Source: CAD feature listing. Evaluate the final solid. Frame: model axes, mm. A direction names the side the tool comes from. Give positions to 0.01 mm unless a question says otherwise; leave off trailing zeros. Loops run counter-clockwise (first coordinate to the right, second up) from the corner with the lowest first, then second, coordinate; pieces in that order, holes last. Notation, with made-up numbers: M 22.5,3.25 L 60.5,3.25 A25 ccw 60.5,17.25 Z; hole C 21.5,88.5 d8. An arc over 180 degrees is marked long. Answer in a Markdown table with one row per item.
```python
from build123d import *

# Parameters (mm, degrees)
SKETCH1_W           = 44.1
SKETCH1_H           = 8
BOSS_EXTRUDE1_DEPTH = 2
SKETCH2_W           = 12
SKETCH2_H           = 2
BOSS_EXTRUDE2_DEPTH = 3
CUT_EXTRUDE1_DEPTH  = 46.097782651
SKETCH4_W           = 32.1
SKETCH4_H           = 2
BOSS_EXTRUDE3_DEPTH = 1
SKETCH7_R           = 2.794
CUT_EXTRUDE3_DEPTH  = 45.382541613
SKETCH8_R           = 1.5875
CUT_EXTRUDE4_DEPTH  = 45.382541613
BOSS_EXTRUDE4_DEPTH = 3


with BuildPart() as part:
    # Sketch1 → Boss-Extrude1 (new body)
    with BuildSketch(Plane(origin=(0, 0, 0), x_dir=(1, 0, 0), z_dir=(0, 1, 0))):
        with Locations((22.05, 0)):
            Rectangle(SKETCH1_W, SKETCH1_H)
    boss_extrude1 = extrude(amount=BOSS_EXTRUDE1_DEPTH)

    # Sketch2 → Boss-Extrude2 (add)
    with BuildSketch(Plane(origin=(0, 2, 0), x_dir=(1, 0, 0), z_dir=(0, 1, 0))):
        with Locations((38.1, 3)):
            Rectangle(SKETCH2_W, SKETCH2_H)
        with Locations((38.1, -3)):
            Rectangle(SKETCH2_W, SKETCH2_H)
    boss_extrude2 = extrude(amount=BOSS_EXTRUDE2_DEPTH)

    # Sketch3 → Cut-Extrude1 (cut, through all)
    with BuildSketch(Plane.XY.offset(4)):
        with BuildLine():
            Line((36.6, 3.5), (36.6, 5))
            Line((36.6, 5), (39.6, 5))
            Line((39.6, 5), (39.6, 3.5))
            ThreePointArc((39.6, 3.5), (38.1, 2), (36.6, 3.5))
        make_face()
    cut_extrude1 = extrude(amount=-CUT_EXTRUDE1_DEPTH, mode=Mode.SUBTRACT)

    # Sketch4 → Boss-Extrude3 (add)
    with BuildSketch(Plane(origin=(0, 2, 0), x_dir=(1, 0, 0), z_dir=(0, 1, 0))):
        with Locations((16.05, -3)):
            Rectangle(SKETCH4_W, SKETCH4_H)
        with Locations((16.05, 3)):
            Rectangle(SKETCH4_W, SKETCH4_H)
    boss_extrude3 = extrude(amount=BOSS_EXTRUDE3_DEPTH)

    # Mirror1: Boss-Extrude1, Boss-Extrude2, Cut-Extrude1, Boss-Extrude3 across plane
    add(boss_extrude1.mirror(Plane(origin=(0, 0, 0), x_dir=(0, 0, 1), z_dir=(1, 0, 0))))
    add(boss_extrude2.mirror(Plane(origin=(0, 0, 0), x_dir=(0, 0, 1), z_dir=(1, 0, 0))))
    add(cut_extrude1.mirror(Plane(origin=(0, 0, 0), x_dir=(0, 0, 1), z_dir=(1, 0, 0))), mode=Mode.SUBTRACT)
    add(boss_extrude3.mirror(Plane(origin=(0, 0, 0), x_dir=(0, 0, 1), z_dir=(1, 0, 0))))

    # Sketch7 → Cut-Extrude3 (cut, through all)
    with BuildSketch(Plane(origin=(0, 2, 0), x_dir=(1, 0, 0), z_dir=(0, 1, 0))):
        Circle(SKETCH7_R)
    extrude(amount=CUT_EXTRUDE3_DEPTH, mode=Mode.SUBTRACT)

    # Sketch8 → Cut-Extrude4 (cut, through all)
    with BuildSketch(Plane(origin=(0, 2, 0), x_dir=(1, 0, 0), z_dir=(0, 1, 0))):
        with Locations(Location((0, 0, 0), (0, 0, 270))):
            Circle(SKETCH8_R)
    extrude(amount=-CUT_EXTRUDE4_DEPTH, mode=Mode.SUBTRACT)

    # Sketch9 → Boss-Extrude4 (add)
    with BuildSketch(Plane(origin=(0, 3, 0), x_dir=(1, 0, 0), z_dir=(0, 1, 0))):
        with BuildLine():
            Line((-2.642429942, -4), (2.642429942, -4))
            ThreePointArc((2.642429942, -4), (0, -4.794), (-2.642429942, -4))
        make_face()
        with BuildLine():
            Line((2.642429942, 4), (-2.642429942, 4))
            ThreePointArc((-2.642429942, 4), (0, 4.794), (2.642429942, 4))
        make_face()
    extrude(amount=-BOSS_EXTRUDE4_DEPTH)


solid = part.part
```
1) Section C-C, the plane x = 17. Return loops of the section in (y, z).
Reply:
| item | result |
|---|---|
| outline | M 0,-4 L 3,-4 L 3,-2 L 2,-2 L 2,2 L 3,2 L 3,4 L 0,4 Z |
2) Section A-A, the plane x = 0. Return loops of the section in (y, z), then the cut area to 3 significant figures.
Reply:
| item | result |
|---|---|
| outline | M 0,-4.79 L 3,-4.79 L 3,-2.79 L 2,-2.79 L 2,-1.59 L 0,-1.59 Z; M 0,1.59 L 2,1.59 L 2,2.79 L 3,2.79 L 3,4.79 L 0,4.79 Z |
| area | 16.8 mm² |
3) Section B-B, the plane z = 0. Return loops of the section in (x, y).
Reply:
| item | result |
|---|---|
| outline | M -44.1,0 L -1.59,0 L -1.59,2 L -44.1,2 Z; M 1.59,0 L 44.1,0 L 44.1,2 L 1.59,2 Z |
4) Pin query (flat end, axial travel): pin 1 Ø4 at (x, z) = (-18.5, -0.5) entering from +Y; pin 2 Ø2.5 at (x, y) = (40.5, 3) entering from +Z; pin 3 Ø2.5 at (x, y) = (-27.5, 2.5) entering from -Z; pin 4 Ø1.5 at (x, y) = (-11.5, 4) entering from -Z. Return the tip coordinate at first contact, or that it passes through.
Reply:
| item | result |
|---|---|
| pin 1 | stops at y = 3 |
| pin 2 | stops at z = 4 |
| pin 3 | stops at z = -4 |
| pin 4 | passes through |
5) Pull-direction query (X, two-part tool) for faces 5 (the flat face through (39.6, 4, 3)), 6 (the flat face through (44.1, 1, 0)), 7 (the flat face through (24, 2, 4)), 8 (the cylindrical face through (-0.966, 1.014, -1.26)); classes: released by +X, released by -X, zero draft, split by the parting line, or undercut.
Reply:
| item | result |
|---|---|
| face 5 | undercut |
| face 6 | released by +X |
| face 7 | zero draft |
| face 8 | undercut |
6) Material intervals for L1, parallel to X at y = 3.6, z = -2.5; L2, parallel to X at y = 1.4, z = 0; L3, parallel to Z at x = -22, y = 2.35, sorted ascending.
Reply:
| item | result |
|---|---|
| L1 | x = -44.1 to -39.6, -36.6 to -32.1, 32.1 to 36.6, 39.6 to 44.1 |
| L2 | x = -44.1 to -1.59, 1.59 to 44.1 |
| L3 | z = -4 to -2, 2 to 4 |
7) Set-up query: faces 1 (the flat face through (24, 2, -4)), 2 (the flat face through (1, 0, -2)), 3 (the flat face through (-36.6, 4, -3)), 4 (the flat face through (-23, 2, -4)). Return all of +Z, -Z, +X, -X, +Y, -Y with unobstructed straight access to the full face (end or side cutting, diameter ignored); none if empty.
Reply:
| item | result |
|---|---|
| face 1 | -Z, +X, +Y, -Y |
| face 2 | +Z, -Z, +X, -X, -Y |
| face 3 | +Z, -Z, +Y |
| face 4 | -Z, -X, +Y, -Y |
